from build123d import *

# Parameters (mm, degrees)
SKETCH1_R          = 32
BASE_FLANGE1_DEPTH = 1.5
SKETCH6_R          = 1.6
CUT_EXTRUDE1_DEPTH = 46.279686395
SKETCH7_W          = 6
SKETCH7_H          = 9
CUT_EXTRUDE2_DEPTH = 46.279686395
FILLET1_R          = 1
SKETCH8_R          = 1.45
CUT_EXTRUDE3_DEPTH = 46.279686395


# Sheet-metal steps are written as plain solids
with BuildPart() as part:
    # Sketch1 → Base-Flange1 (new body)
    with BuildSketch(Plane(origin=(0, 0, 0), x_dir=(1, 0, 0), z_dir=(0, 1, 0))):
        with Locations(Location((0, 0, 0), (0, 0, 270))):
            Circle(SKETCH1_R)
    extrude(amount=-BASE_FLANGE1_DEPTH)

    # Sketch6 → Cut-Extrude1 (cut, through all)
    with BuildSketch(Plane(origin=(0, 0, 0), x_dir=(1, 0, 0), z_dir=(0, 1, 0))):
        with Locations(Location((-28, 0, 0), (0, 0, 270))):
            Circle(SKETCH6_R)
        with Locations(Location((14, 24.248711306, 0), (0, 0, 270))):
            Circle(SKETCH6_R)
        with Locations(Location((14, -24.248711306, 0), (0, 0, 270))):
            Circle(SKETCH6_R)
    extrude(amount=-CUT_EXTRUDE1_DEPTH, mode=Mode.SUBTRACT)

    # Sketch7 → Cut-Extrude2 (cut, through all)
    with BuildSketch(Plane(origin=(0, 0, 0), x_dir=(1, 0, 0), z_dir=(0, 1, 0))):
        with Locations((-21, 0)):
            Rectangle(SKETCH7_W, SKETCH7_H)
    extrude(amount=-CUT_EXTRUDE2_DEPTH, mode=Mode.SUBTRACT)

    # Fillet1
    fillet1_edges = [part.edges().sort_by_distance(p)[0] for p in [
        (-18, -0.75, -4.5),
        (-18, -0.75, 4.5),
        (-24, -0.75, 4.5),
        (-24, -0.75, -4.5),
    ]]
    fillet(fillet1_edges, radius=FILLET1_R)

    # Sketch8 → Cut-Extrude3 (cut, through all)
    with BuildSketch(Plane.XZ.offset(1.5)):
        with Locations(Location((2.55, -14.75, 0), (0, 0, 270))):
            Circle(SKETCH8_R)
        with Locations(Location((2.55, 14.75, 0), (0, 0, 270))):
            Circle(SKETCH8_R)
        with Locations(Location((-20.55, 14.75, 0), (0, 0, 270))):
            Circle(SKETCH8_R)
        with Locations(Location((-20.55, -14.75, 0), (0, 0, 270))):
            Circle(SKETCH8_R)
    extrude(amount=-CUT_EXTRUDE3_DEPTH, mode=Mode.SUBTRACT)


solid = part.part
Here's how the part is built. I have some questions about the finished solid (model axes, mm). A direction names the side the tool comes from. Round coordinates to 2 decimals unless told otherwise and drop trailing zeros. Write each loop counter-clockwise with the first axis right and the second up, starting at its lowest first coordinate (ties: lowest second). Pieces come first, ordered by that corner, then holes.
1. For faces 1 (the flat face through (-24, -1, 0)), 2 (the flat face through (0, 0, 0)), which set-ups out of +Z, -Z, +X, -X, +Y, -Y let a thin tool reach every point of the face, with its end or its side?
2. Suppose I cut it at A-A (y = -0.75). State how many separate pieces and enclosed holes the cut face has, and give its area (3 significant figures).
3. Will these pins go through, and if not, where does the flat tip stop? pin 1 Ø0.8 at (y, z) = (-1, -0.5) entering from -X; pin 2 Ø3.5 at (x, z) = (2.55, 14.75) entering from +Y; pin 3 Ø1.7 at (x, z) = (-20.55, 14.75) entering from +Y.
4. Suppose I cut it at C-C (x = 14). List the corners of the cut face in (y, z) for me.
5. Suppose I cut it at D-D (x = -28). List the corners of the cut face in (y, z) for me, and give its area (3 significant figures).
6. Suppose I cut it at B-B (z = -14.75). List the corners of the cut face in (x, y) for me, and give its area (3 significant figures).
7. I need wall thicknesses on L1, parallel to X at y = -0.6, z = 0; L2, parallel to X at y = -1, z = 14.75; L3, parallel to X at y = -1.1, z = 24. Which ranges of each line are inside material? Lowest first, please.
Answer sheet:
1. face 1: +Y, -Y
1. face 2: +Z, -Z, +X, -X, +Y
2. separate pieces: 1
2. enclosed holes: 8
2. area: 3,110 mm2
3. pin 1: stops at x = -32
3. pin 2: stops at y = 0
3. pin 3: passes through
4. outline: (-1.5, -28.77) - (0, -28.77) - (0, -25.85) - (-1.5, -25.85) - close; (-1.5, -22.65) - (0, -22.65) - (0, 22.65) - (-1.5, 22.65) - close; (-1.5, 25.85) - (0, 25.85) - (0, 28.77) - (-1.5, 28.77) - close
5. outline: (-1.5, -15.49) - (0, -15.49) - (0, -1.6) - (-1.5, -1.6) - close; (-1.5, 1.6) - (0, 1.6) - (0, 15.49) - (-1.5, 15.49) - close
5. area: 41.7 mm2
6. outline: (-28.4, -1.5) - (-22, -1.5) - (-22, 0) - (-28.4, 0) - close; (-19.1, -1.5) - (1.1, -1.5) - (1.1, 0) - (-19.1, 0) - close; (4, -1.5) - (28.4, -1.5) - (28.4, 0) - (4, 0) - close
6. area: 76.5 mm2
7. L1: x = -32 to -29.6, -26.4 to -24, -18 to 32
7. L2: x = -28.4 to -22, -19.1 to 1.1, 4 to 28.4
7. L3: x = -21.17 to 12.42, 15.58 to 21.17
